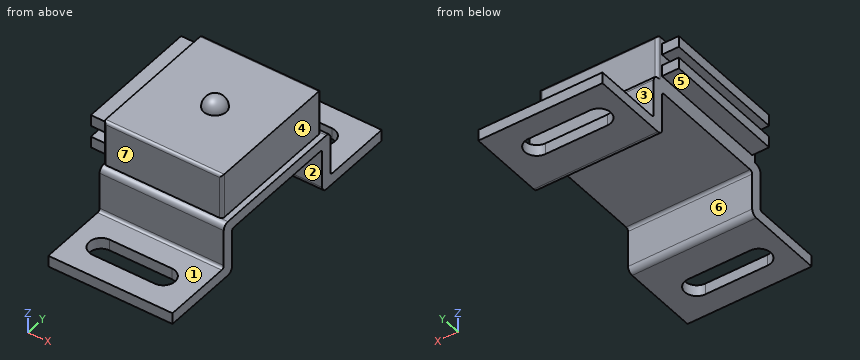
Autodesk Inventor part; units mm, degrees
ref_plane "magnet_dummy_XY" through (0, 0, 0) normal (0, 0, 1) x (1, 0, 0)
ref_plane "magnet_dummy_YZ" through (0, 0, 0) normal (1, 0, 0) x (0, 1, 0)
ref_plane "magnet_dummy_ZX" through (0, 0, 0) normal (0, 1, 0) x (0, 0, 1)
sketch "Sketch_1" plane through (0, 0, 0) normal (1, 0, 0) x (0, 1, 0)
  arc A0 (-11.5, 0) -> (-12, -0.5) centre (-11.5, -0.5) ccw
  line L0 (-12, -0.5) -> (-12, -8)
  arc A1 (-12, -8) -> (-13, -9) centre (-12, -9) ccw
  line L1 (-13, -9) -> (-13, -15.5)
  arc A2 (-13.5, -16) -> (-13, -15.5) centre (-13.5, -15.5) ccw
  line L2 (-13.5, -16) -> (-25.5, -16)
  line L3 (-25.5, -16) -> (-25.5, -18)
  line L4 (-25.5, -18) -> (-12, -18)
  arc A3 (-12, -18) -> (-11, -17) centre (-12, -17) ccw
  line L5 (-11, -17) -> (-11, -10.5)
  arc A4 (-10.5, -10) -> (-11, -10.5) centre (-10.5, -10.5) ccw
  line L6 (-10.5, -10) -> (10.5, -10)
  arc A5 (11, -10.5) -> (10.5, -10) centre (10.5, -10.5) ccw
  line L7 (11, -10.5) -> (11, -17)
  arc A6 (11, -17) -> (12, -18) centre (12, -17) ccw
  line L8 (12, -18) -> (25.5, -18)
  line L9 (25.5, -18) -> (25.5, -16)
  line L10 (25.5, -16) -> (13.5, -16)
  arc A7 (13, -15.5) -> (13.5, -16) centre (13.5, -15.5) ccw
  line L11 (13, -15.5) -> (13, -9)
  arc A8 (13, -9) -> (12, -8) centre (12, -9) ccw
  line L12 (12, -8) -> (12, -0.5)
  arc A9 (12, -0.5) -> (11.5, 0) centre (11.5, -0.5) ccw
  line L13 (11.5, 0) -> (-11.5, 0)
extrude "Extrusion1" add sketch "Sketch_1" along normal mid plane 22
sketch "Sketch_2" plane through (0, 0, 0) normal (0, 0, 1) x (1, 0, 0)
  line L0 (10, 12) -> (10, -12)
  line L1 (10, -12) -> (11, -12)
  line L2 (11, -12) -> (11, 12)
  line L3 (11, 12) -> (10, 12)
extrude "Extrusion2" cut sketch "Sketch_2" against normal blind 8
sketch "Sketch_3" plane through (0, 0, 0) normal (0, 0, 1) x (1, 0, 0)
  line L0 (50, 0) -> (-50, 0)
  arc A0 (2, 0) -> (-2, 0) centre (0, 0) ccw
  line L1 (2, 0) -> (-2, 0)
revolve "Revolution1" add sketch "Sketch_3" angle 360 about axis through (50, 0, 0) along (1, 0, 0)
sketch "Sketch_6" plane through (0, 0, 0) normal (0, 0, 1) x (1, 0, 0)
  line L0 (-24, 24) -> (-24, -24)
  line L1 (-24, -24) -> (24, -24)
  line L2 (24, -24) -> (24, 24)
  line L3 (24, 24) -> (-24, 24)
  line L4 (-11, 11.5) -> (-11, -11.5)
  arc A0 (-11, -11.5) -> (-10.5, -12) centre (-10.5, -11.5) ccw
  line L5 (-10.5, -12) -> (9.5, -12)
  arc A1 (9.5, -12) -> (10, -11.5) centre (9.5, -11.5) ccw
  line L6 (10, -11.5) -> (10, 11.5)
  arc A2 (10, 11.5) -> (9.5, 12) centre (9.5, 11.5) ccw
  line L7 (9.5, 12) -> (-10.5, 12)
  arc A3 (-10.5, 12) -> (-11, 11.5) centre (-10.5, 11.5) ccw
extrude "Extrusion3" cut sketch "Sketch_6" against normal blind 8
sketch "Sketch_4" plane through (-11, 0, 0) normal (1, 0, 0) x (0, 0, -1)
  line L0 (1, 11) -> (1, -11)
  line L1 (1, -11) -> (3, -11)
  line L2 (3, -11) -> (3, 11)
  line L3 (3, 11) -> (1, 11)
extrude "Extrusion4" add sketch "Sketch_4" against normal blind 3
sketch "Sketch_5" plane through (-11, 0, 0) normal (1, 0, 0) x (0, 0, -1)
  line L0 (5, -11) -> (7, -11)
  line L1 (7, -11) -> (7, 11)
  line L2 (7, 11) -> (5, 11)
  line L3 (5, 11) -> (5, -11)
extrude "Extrusion5" add sketch "Sketch_5" against normal blind 3
sketch "Sketch_7" plane through (0, 0, 0) normal (0, 0, 1) x (1, 0, 0)
  arc A0 (-6, 21.6) -> (-6, 17.4) centre (-6, 19.5) ccw
  line L0 (-6, 17.4) -> (5, 17.4)
  arc A1 (5, 17.4) -> (5, 21.6) centre (5, 19.5) ccw
  line L1 (5, 21.6) -> (-6, 21.6)
extrude "Extrusion6" cut sketch "Sketch_7" against normal blind 20
sketch "Sketch_8" plane through (0, 0, 0) normal (0, 0, 1) x (1, 0, 0)
  arc A0 (-6, -17.4) -> (-6, -21.6) centre (-6, -19.5) ccw
  line L0 (-6, -21.6) -> (5, -21.6)
  arc A1 (5, -21.6) -> (5, -17.4) centre (5, -19.5) ccw
  line L1 (5, -17.4) -> (-6, -17.4)
extrude "Extrusion7" cut sketch "Sketch_8" against normal blind 20
ref_plane "magnet_dummy_XY" through (0, 0, 0) normal (0, 0, 1) x (1, 0, 0)
ref_plane "magnet_dummy_YZ" through (0, 0, 0) normal (1, 0, 0) x (0, 1, 0)
ref_plane "magnet_dummy_ZX" through (0, 0, 0) normal (0, 1, 0) x (0, 0, 1)
ref_plane "to_ap_plate_XY" through (-9.1, 26, 0) normal (0, 0, -1) x (1, 0, 0)
ref_plane "to_ap_plate_YZ" through (-9.1, 26, 0) normal (1, 0, 0) x (0, -1, 0)
ref_plane "to_ap_plate_ZX" through (-9.1, 26, 0) normal (0, -1, 0) x (0, 0, -1)
ref_plane "to_door_side_plate_XY" through (-14, 0, -6) normal (1, 0, 0) x (0, 0, -1)
ref_plane "to_door_side_plate_YZ" through (-14, 0, -6) normal (0, 0, -1) x (0, 1, 0)
ref_plane "to_door_side_plate_ZX" through (-14, 0, -6) normal (0, 1, 0) x (1, 0, 0)
ref_plane "to_ap_plate1_XY" through (-1, 19.5, -18) normal (0, 0, 1) x (1, 0, 0)
ref_plane "to_ap_plate1_YZ" through (-1, 19.5, -18) normal (1, 0, 0) x (0, 1, 0)
ref_plane "to_ap_plate1_ZX" through (-1, 19.5, -18) normal (0, 1, 0) x (0, 0, 1)
ref_plane "to_ap_plate2_XY" through (-1, -19.5, -18) normal (0, 0, 1) x (1, 0, 0)
ref_plane "to_ap_plate2_YZ" through (-1, -19.5, -18) normal (1, 0, 0) x (0, 1, 0)
ref_plane "to_ap_plate2_ZX" through (-1, -19.5, -18) normal (0, 1, 0) x (0, 0, 1)
ref_plane "x1_XY" through (-9.2, 26, -15) normal (0, 0, -1) x (1, 0, 0)
ref_plane "x1_YZ" through (-9.2, 26, -15) normal (1, 0, 0) x (0, -1, 0)
ref_plane "x1_ZX" through (-9.2, 26, -15) normal (0, -1, 0) x (0, 0, -1)
ref_plane "x2_XY" through (-9.2, -26, -15) normal (0, 0, -1) x (1, 0, 0)
ref_plane "x2_YZ" through (-9.2, -26, -15) normal (1, 0, 0) x (0, -1, 0)
ref_plane "x2_ZX" through (-9.2, -26, -15) normal (0, -1, 0) x (0, 0, -1)
ref_plane "magnet_to_dummy2_XY" through (0, 0, -15) normal (0, 0, 1) x (1, 0, 0)
ref_plane "magnet_to_dummy2_YZ" through (0, 0, -15) normal (1, 0, 0) x (0, 1, 0)
ref_plane "magnet_to_dummy2_ZX" through (0, 0, -15) normal (0, 1, 0) x (0, 0, 1)
ref_plane "xy1_XY" through (-9.5, -26, 0) normal (0, 0, 1) x (1, 0, 0)
ref_plane "xy1_YZ" through (-9.5, -26, 0) normal (1, 0, 0) x (0, 1, 0)
ref_plane "xy1_ZX" through (-9.5, -26, 0) normal (0, 1, 0) x (0, 0, 1)
ref_plane "x22_XY" through (-9.1, -26, -7.5) normal (0, 0, -1) x (1, 0, 0)
ref_plane "x22_YZ" through (-9.1, -26, -7.5) normal (1, 0, 0) x (0, -1, 0)
ref_plane "x22_ZX" through (-9.1, -26, -7.5) normal (0, -1, 0) x (0, 0, -1)
ref_plane "to_ap_platexxx_XY" through (-9.1, 26, 0) normal (0, 0, -1) x (1, 0, 0)
ref_plane "to_ap_platexxx_YZ" through (-9.1, 26, 0) normal (1, 0, 0) x (0, -1, 0)
ref_plane "to_ap_platexxx_ZX" through (-9.1, 26, 0) normal (0, -1, 0) x (0, 0, -1)
ref_plane "to_ap_plate3_XY" through (-1, -19.5, -18) normal (0, 0, 1) x (1, 0, 0)
ref_plane "to_ap_plate3_YZ" through (-1, -19.5, -18) normal (1, 0, 0) x (0, 1, 0)
ref_plane "to_ap_plate3_ZX" through (-1, -19.5, -18) normal (0, 1, 0) x (0, 0, 1)
ref_plane "magnet_to_plate_XY" through (0, 19.5, -18) normal (1, 0, 0) x (0, 0, -1)
ref_plane "magnet_to_plate_YZ" through (0, 19.5, -18) normal (0, 0, -1) x (0, 1, 0)
ref_plane "magnet_to_plate_ZX" through (0, 19.5, -18) normal (0, 1, 0) x (1, 0, 0)
ref_plane "to_plate_XY" through (-9.1, 26, -15) normal (0, 0, -1) x (1, 0, 0)
ref_plane "to_plate_YZ" through (-9.1, 26, -15) normal (1, 0, 0) x (0, -1, 0)
ref_plane "to_plate_ZX" through (-9.1, 26, -15) normal (0, -1, 0) x (0, 0, -1)
ref_plane "to_pwf_bolt_XY" through (-9.1, 26, 0) normal (0, 0, -1) x (1, 0, 0)
ref_plane "to_pwf_bolt_YZ" through (-9.1, 26, 0) normal (1, 0, 0) x (0, -1, 0)
ref_plane "to_pwf_bolt_ZX" through (-9.1, 26, 0) normal (0, -1, 0) x (0, 0, -1)
ref_plane "to_pwf_bolt_1_XY" through (-9.1, -26, 0) normal (0, 0, -1) x (1, 0, 0)
ref_plane "to_pwf_bolt_1_YZ" through (-9.1, -26, 0) normal (1, 0, 0) x (0, -1, 0)
ref_plane "to_pwf_bolt_1_ZX" through (-9.1, -26, 0) normal (0, -1, 0) x (0, 0, -1)
ref_plane "washer_1_XY" through (-9.2, 26, 0) normal (0, 0, -1) x (1, 0, 0)
ref_plane "washer_1_YZ" through (-9.2, 26, 0) normal (1, 0, 0) x (0, -1, 0)
ref_plane "washer_1_ZX" through (-9.2, 26, 0) normal (0, -1, 0) x (0, 0, -1)
ref_plane "washer_2_XY" through (-9.2, -26, 0) normal (0, 0, -1) x (1, 0, 0)
ref_plane "washer_2_YZ" through (-9.2, -26, 0) normal (1, 0, 0) x (0, -1, 0)
ref_plane "washer_2_ZX" through (-9.2, -26, 0) normal (0, -1, 0) x (0, 0, -1)
ref_plane "pmf_1_XY" through (-9.2, 26, 0.8) normal (0, 0, -1) x (1, 0, 0)
ref_plane "pmf_1_YZ" through (-9.2, 26, 0.8) normal (1, 0, 0) x (0, -1, 0)
ref_plane "pmf_1_ZX" through (-9.2, 26, 0.8) normal (0, -1, 0) x (0, 0, -1)
ref_plane "pmf_2_XY" through (-9.2, -26, 0.8) normal (0, 0, -1) x (1, 0, 0)
ref_plane "pmf_2_YZ" through (-9.2, -26, 0.8) normal (1, 0, 0) x (0, -1, 0)
ref_plane "pmf_2_ZX" through (-9.2, -26, 0.8) normal (0, -1, 0) x (0, 0, -1)
properties part number "HMEN5-5-magnet"
Verification items for the finished model (mm, model axes). Face numbers are marked on the shaded views. A direction names the side the tool comes from. Give positions to 0.01 mm unless a question says otherwise; leave off trailing zeros. Order: outer loops, then holes, each group sorted by start corner. A loop starts at its lowest first (then second) coordinate and runs counter-clockwise, first axis right, second up. Notation, with made-up numbers: M 20.25,29 L 70.25,29 A13 cw 70.25,47 Z; hole C 66,53.25 d8. An arc over 180 degrees is marked long. Answer as a JSON object with one key per item and string values. Group by question number.
1) Scan lines: line 1 along Y through (x, z) = (1, -16.5); line 2 along Y through (x, z) = (6, -10.5); line 3 along X through (y, z) = (7, -1.75). Record each from-to range of solid material in increasing order. Write a range as [from, to].
2) Cross-section at D-D (x = -2.75). Give the number of separate pieces and of enclosed holes in the cut face, then the cut area to 3 significant figures.
3) Cross-section at A-A (z = -16.5). Enter the section's corners in (x, y), then the cut area to 3 significant figures.
4) Cross-section at C-C (y = 19.5). Enter the section's corners in (x, z), then the cut area to 3 significant figures.
5) Depth check by flat-ended pin: pin 1 Ø0.6 at (x, y) = (-10.5, -12) entering from +Z; pin 2 Ø10.5 at (x, y) = (5, 3.5) entering from -Z; pin 3 Ø0.6 at (x, z) = (-13, -6.5) entering from -Y. Enter the tip coordinate at first touch or a pass-through.
6) Access from +Z, -Z, +X, -X, +Y, -Y to the whole of each face (thin tool, end or side, straight path). Record for the marked faces 1, 2, 3 and 4.
7) Cross-section at B-B (x = -12). Enter the section's corners in (y, z).
8) Mould release check, pull along Y, two halves, no side actions. Record for the marked faces 5, 6 and 7: released by +Y, released by -Y, zero draft, split by the parting line, or undercut.
Result sheet:
{
 "1": {"line 1": "y = [-25.5, -21.6], [-17.4, -11], [11, 17.4], [21.6, 25.5]", "line 2": "y = [-13, -11], [11, 13]", "line 3": "x = [-14, 10]"},
 "2": {"separate pieces": "3", "enclosed holes": "0", "area": "308 mm2"},
 "3": {"outline": "M -11,-25.5 L 11,-25.5 L 11,-11 L -11,-11 Z; M -11,11 L 11,11 L 11,25.5 L -11,25.5 Z; hole M -6,-21.6 L 5,-21.6 A2.1 ccw 5,-17.4 L -6,-17.4 A2.1 ccw Z; hole M -6,17.4 L 5,17.4 A2.1 ccw 5,21.6 L -6,21.6 A2.1 ccw Z", "area": "518 mm2"},
 "4": {"outline": "M -11,-18 L -8.1,-18 L -8.1,-16 L -11,-16 Z; M 7.1,-18 L 11,-18 L 11,-16 L 7.1,-16 Z", "area": "13.6 mm2"},
 "5": {"pin 1": "stops at z = -0.04", "pin 2": "stops at z = -10", "pin 3": "stops at y = -11"},
 "6": {"face 1": "+Z, +X, -X, -Y", "face 2": "-Z, +X, -X", "face 3": "+Z, +X, -X, +Y", "face 4": "+Z, +X, +Y, -Y"},
 "7": {"outline": "M -11,-7 L 11,-7 L 11,-5 L -11,-5 Z; M -11,-3 L 11,-3 L 11,-1 L -11,-1 Z"},
 "8": {"face 5": "zero draft", "face 6": "undercut", "face 7": "released by -Y"}
}
